Here's the drawing with two shaded views (mm, measured from the low corner). I have some questions. A direction names the side the tool comes from. Give positions to 0.01 mm unless a question says otherwise; leave off trailing zeros. Write each loop counter-clockwise with the first axis right and the second up, starting at its lowest first coordinate (ties: lowest second). Pieces come first, ordered by that corner, then holes. Notation, with made-up numbers: M 50,-8 L 81,-8 A14 cw 81,14 Z; hole C -36,9 d5. An arc over 180 degrees is marked long. Answer as a JSON object with one key per item and string values. Group by question number.
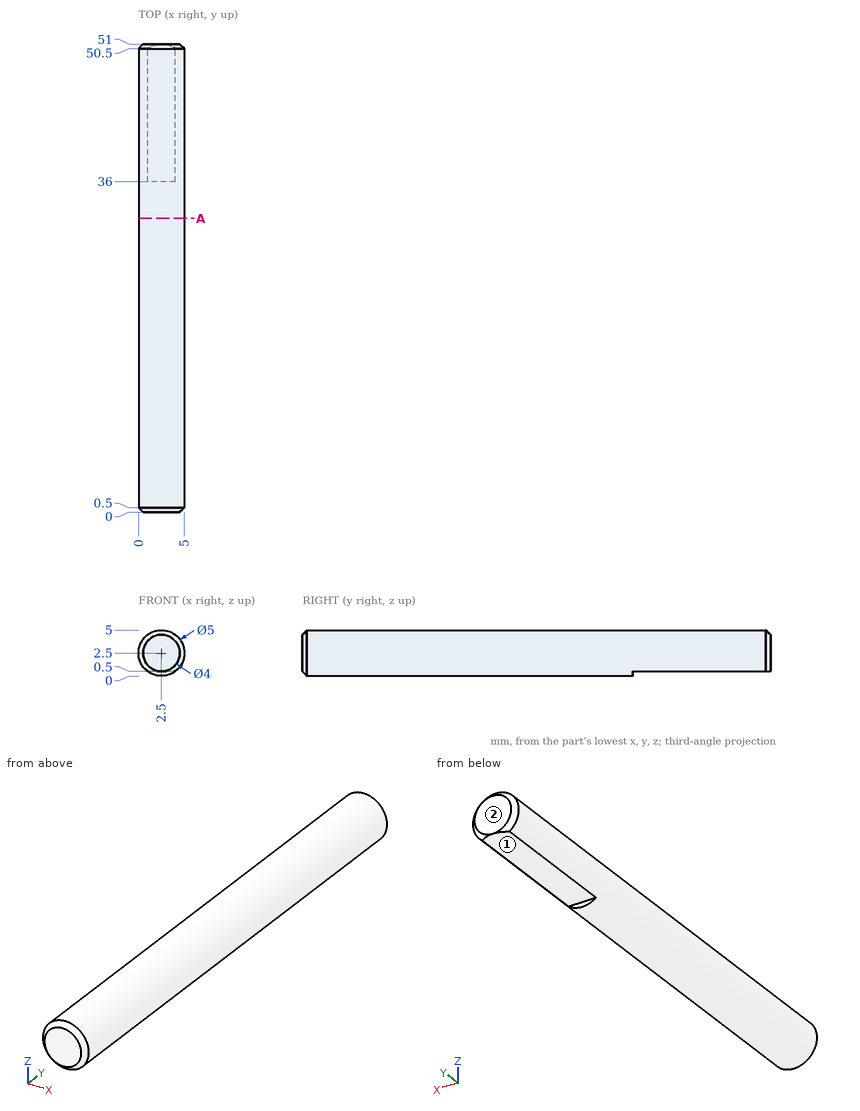
1) Please list where these lines run through material, in increasing order: line 1 along Z through (x, y) = (2.6, 13.5); line 2 along X through (y, z) = (12, 2.3); line 3 along Y through (x, z) = (0.6, 3.4). Write a range as from..to.
2) If we section it at A-A, the plane y = 32: List the corners of the cut face in (x, z) for me.
3) For the marked faces 1 and 2, which set-ups out of +Z, -Z, +X, -X, +Y, -Y let a thin tool reach every point of the face, with its end or its side?
4) I'm going to push flat-ended pins straight in: pin 1 (0.5 mm diameter, centred on x = 2.5, z = 0, fed in from +Y); pin 2 (1 mm diameter, centred on y = 34.5, z = 4, fed in from -X). Where does each tip first touch, or does it pass through?
Taken from the geometry:
{
 "1": {"line 1": "0..5", "line 2": "0.01..4.99", "line 3": "0.1..50.9"},
 "2": {"outline": "C 2.5,2.5 d5"},
 "3": {"face 1": "-Z, +X, -X, +Y", "face 2": "+Z, -Z, +X, -X, +Y"},
 "4": {"pin 1": "y = 36", "pin 2": "x = 0.21"}
}
